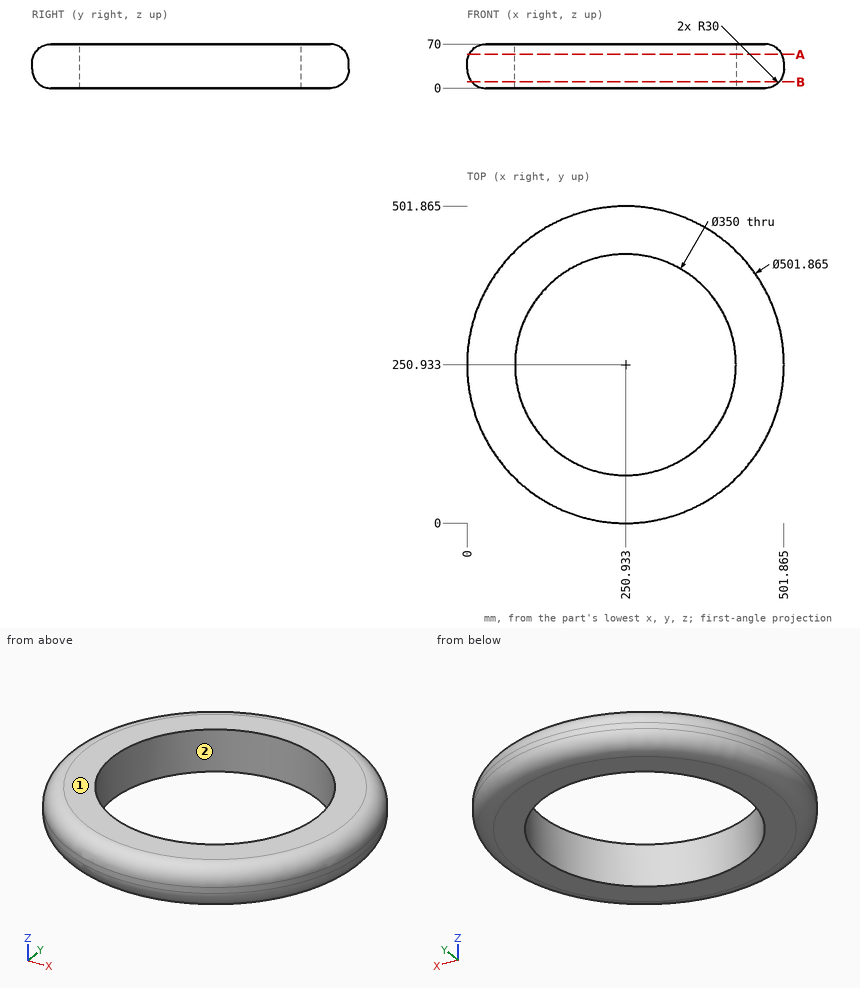
Job drawing, mm, ordinate dimensions from the low corner. One solid piece. Round coordinates to 2 decimals unless told otherwise and drop trailing zeros. Write each loop counter-clockwise with the first axis right and the second up, starting at its lowest first coordinate (ties: lowest second). Pieces come first, ordered by that corner, then holes.
1) Band-saw the part on A-A, the plane z = 53.5. List the corners of the cut face in (x, y).
2) Mould opens along X. For the marked faces 1 and 2 say: +X half, -X half, draft (parallel to the pull), parting line (faces both ways), or undercut.
3) Pin check, flat tips, straight feed: pin 1 (12 mm diameter, centred on x = 224.5, z = 10.5, fed in from -Y); pin 2 (4 mm diameter, centred on y = 136, z = 52.5, fed in from +X); pin 3 (10 mm diameter, centred on y = 304.5, z = 30, fed in from -X) (1 decimal). Stop position of each tip, or through.
4) Band-saw the part on B-B, the plane z = 10. List the corners of the cut face in (x, y).
5) Drill centre lines: probe 1 along Y at (x, z) = (264, 41); probe 2 along Y at (x, z) = (331.5, 65.5) (1 decimal); probe 3 along X at (y, z) = (133, 58) (1 decimal). Where is each one in solid material? Low to high.
Ans:
1. outline: circle Ø495.45 at (250.93, 250.93); hole circle Ø350 at (250.93, 250.93)
2. face 1: draft
2. face 2: undercut
3. pin 1: stops at y = 4.56
3. pin 2: stops at x = 472.34
3. pin 3: stops at x = 4.7
4. outline: circle Ø486.59 at (250.93, 250.93); hole circle Ø350 at (250.93, 250.93)
5. probe 1: y = 0.36 to 76.42, 425.44 to 501.51
5. probe 2: y = 28.3 to 95.6, 406.3 to 473.5
5. probe 3: x = 36.3 to 121.6, 380.2 to 465.6
